Design review of the part built by this model. Coordinates are the model's own, in mm. A direction names the side the tool comes from. Round coordinates to 2 decimals unless told otherwise and drop trailing zeros. Order: outer loops, then holes, each group sorted by start corner. A loop starts at its lowest first (then second) coordinate and runs counter-clockwise, first axis right, second up.
from build123d import *

# Parameters (mm, degrees)
BOSS_EXTRUDE1_DEPTH = 3.85
CHAMFER1_SIZE       = 1


with BuildPart() as part:
    # Sketch1 → Boss-Extrude1 (new body)
    with BuildSketch(Plane.XY):
        Polygon((25, 0), (19.7125, 9.158218645), (15.382372981, 6.658218645), (13.457372981, 9.99241645), (17.7875, 12.49241645), (12.5, 21.650635095), (-12.5, 21.650635095), (-17.7875, 12.49241645), (-13.457372981, 9.99241645), (-15.382372981, 6.658218645), (-19.7125, 9.158218645), (-25, 0), (-12.5, -21.650635095), (-1.925, -21.650635095), (-1.925, -16.650635095), (1.925, -16.650635095), (1.925, -21.650635095), (12.5, -21.650635095), align=None)
    extrude(amount=BOSS_EXTRUDE1_DEPTH)

    # Chamfer1
    chamfer1_edges = [part.edges().sort_by_distance(p)[0] for p in [
        (1.925, -21.650635095, 1.925),
        (-1.925, -21.650635095, 1.925),
        (-19.7125, 9.158218645, 1.925),
        (-17.7875, 12.49241645, 1.925),
        (17.7875, 12.49241645, 1.925),
        (19.7125, 9.158218645, 1.925),
    ]]
    chamfer(chamfer1_edges, length=CHAMFER1_SIZE)


solid = part.part
1) Take a section at B-B on x = -1. Give the boundary of the cut face in (y, z).
Results:
outline: (-16.65, 0) - (21.65, 0) - (21.65, 3.85) - (-16.65, 3.85) - close
2) To check wall thickness, follow line 1 along X through (y, z) = (12, 2.35); line 2 along X through (y, z) = (7, 3.2); line 3 along Y through (x, z) = (-20.5, 0.45). State the ranges of each line that lie inside material, in increasing order.
Results:
line 1: x = -16.92 to 16.92
line 2: x = -20.96 to -15.97, -15.19 to 15.19, 15.97 to 20.96
line 3: y = -7.79 to 7.79
3) Take a section at A-A on z = 0.6. Give the boundary of the cut face in (x, y) (1 decimal), plus the area to 3 significant figures.
Results:
outline: (-25, 0) - (-12.5, -21.7) - (-2.9, -21.7) - (-1.9, -20.7) - (-1.9, -16.7) - (1.9, -16.7) - (1.9, -20.7) - (2.9, -21.7) - (12.5, -21.7) - (25, 0) - (20.2, 8.3) - (18.8, 8.7) - (15.4, 6.7) - (13.5, 10) - (16.9, 12) - (17.3, 13.4) - (12.5, 21.7) - (-12.5, 21.7) - (-17.3, 13.4) - (-16.9, 12) - (-13.5, 10) - (-15.4, 6.7) - (-18.8, 8.7) - (-20.2, 8.3) - close
area: 1,560 mm2
4) For faces 1 (the face through (-17.102, 12.666, 1.898)), 2 (the face through (1.925, -19, 2)), 3 (the face through (14.433, 8.302, 1.898)), 4 (the face through (17.107, 12.685, 1.898)), list the 3-axis set-ups (+Z, -Z, +X, -X, +Y, -Y) from which the entire face can be reached by the end or side of a thin tool; tool diameter is ignored.
Results:
face 1: +Z, -Z, -X
face 2: +Z, -Z, -Y
face 3: +Z, -Z
face 4: +Z, -Z, +X
5) The part is to be moulded in two halves that separate along Y. For faces 5 (the face through (18.66, -10.98, 1.9)), 6 (the face through (0, 0, 0)), 7 (the face through (14.927, 17.446, 1.898)), 8 (the face through (-15.2, 11, 1.9)), say which applies: released by +Y, released by -Y, zero draft, split by the parting line, or undercut.
Results:
face 5: released by -Y
face 6: zero draft
face 7: released by +Y
face 8: undercut
6) Clearance check with flat-ended pins moving along their axes: P1, Ø2, axis at y = 13, z = 0.5, coming from the -X side; P2, Ø1.9, axis at y = -18.5, z = 3, coming from the -X side. State where each tip first meets the part, or that it passes through.
Results:
P1: stops at x = -17.29
P2: stops at x = -14.87
7) Take a section at C-C on y = -2. Give the boundary of the cut face in (x, z).
Results:
outline: (-23.85, 0) - (23.85, 0) - (23.85, 3.85) - (-23.85, 3.85) - close
